The model under review builds one solid part; all positions refer to its coordinate system, in mm. A direction names the side the tool comes from. Coordinates: 2 decimals unless noted, no trailing zeros. Loops run counter-clockwise (first coordinate to the right, second up) from the corner with the lowest first, then second, coordinate; pieces in that order, holes last. Notation, with made-up numbers: M 64,68 L 71,68 A20 cw 71,93 Z; hole C 23,-18 d2. An arc over 180 degrees is marked long. Return JSON: item names as keys, results as strings.
Autodesk Fusion 360 part; units mm, degrees
sketch "スケッチ1" plane through (0, 0, 0) normal (0, 0, 1) x (1, 0, 0)
  line L0 (-19, 20) -> (19, 20)
  line L1 (19, 20) -> (19, 0)
  line L2 (19, 0) -> (-19, 0)
  line L3 (-19, 0) -> (-19, 20)
  dimension "d1" = 38
  dimension "d2" = 20
extrude "押し出し1" add sketch "スケッチ1" along normal blind 16
sketch "スケッチ2" plane through (0, 0, 16) normal (0, 0, 1) x (-1, 0, 0)
  line L0 (19, 0) -> (-19, 0)
  line L1 (-19, 0) -> (-19, -20)
  line L2 (-19, -20) -> (19, -20)
  line L3 (19, -20) -> (19, 0)
  line L4 (8, 0) -> (-8, 0)
  line L5 (-8, 0) -> (-8, -10)
  line L6 (-8, -10) -> (-15, -10)
  line L7 (-15, -10) -> (-15, -20)
  line L8 (15, -20) -> (15, -10)
  line L9 (15, -10) -> (8, -10)
  line L10 (8, -10) -> (8, 0)
  line L11 (14, -6) -> (-14, -6)
  point P0 (0, -6)
  dimension "d5" = 16
  dimension "d6" = 4
  dimension "d7" = 4
  dimension "d8" = 10
  dimension "d9" = 6
  dimension "d10" = 28
extrude "押し出し2" cut sketch "スケッチ2" against normal blind 11.5 contours L0 L4 L5 L10 L11 | L2 L5 L6 L7 L8 L9 L10 L11
hole "穴1" at (-14, 6, 16) at (14, 6, 16) direction (0, 0, -1) diameter 3 depth 10 tip angle 118
thread "ねじ1"
fillet "フィレット1" radius 4 2 edges at (19, 0, 8) (-19, 0, 8)
1. Add section A-A on y = 11.25. Give the boundary of the cut face in (x, z).
Check values:
{"outline": "M -19,0 L 19,0 L 19,16 L 15,16 L 15,4.5 L -15,4.5 L -15,16 L -19,16 Z"}
2. To check wall thickness, follow line 1 (X direction, y = 6, z = 10.25); line 2 (Y direction, x = 14, z = 10.5); line 3 (X direction, y = 8.75, z = 9.75). State the ranges of each line that lie inside material, in increasing order.
Check values:
{"line 1": "-19 to -15.5, -12.5 to -8, 8 to 12.5, 15.5 to 19", "line 2": "0 to 4.5, 7.5 to 10", "line 3": "-19 to -8, 8 to 19"}
3. The part is to be moulded in two halves that separate along Y. For faces 4 (the face through (14.22, 5.86, 5.255)), 5 (the face through (-13.1, 7.2, 10.9)), 6 (the face through (-12, 10, 10)), 7 (the face through (15, 8, 16)), say which applies: released by +Y, released by -Y, zero draft, split by the parting line, or undercut.
Check values:
{"face 4": "undercut", "face 5": "undercut", "face 6": "released by +Y", "face 7": "zero draft"}
4. Insertion check: pin 1 Ø7.5 at (x, z) = (11, 10.5) entering from +Y; pin 2 Ø6 at (x, y) = (7, 14.5) entering from +Z. Each pin has a flat end and moves straight along its axis. Give the tip position at first contact, or say it passes through.
Check values:
{"pin 1": "y = 10", "pin 2": "z = 4.5"}
5. Machinability: for faces 1 (the face through (-17.859, 1.203, 8.112)), 2 (the face through (8, 5, 10)), 3 (the face through (11, 10, 10)), which of the approach directions +Z, -Z, +X, -X, +Y, -Y give a long, thin tool a straight path to every point of the face, cutting with its end or side? Answer none if there is none.
Check values:
{"face 1": "+Z, -Z, -X, -Y", "face 2": "+Z, +Y, -Y", "face 3": "+Z, +Y"}
6. Add section B-B on x = -8.5. Give the boundary of the cut face in (y, z), plus the area to 3 significant figures.
Check values:
{"outline": "M 0,0 L 20,0 L 20,4.5 L 10,4.5 L 10,16 L 0,16 Z", "area": "205 mm²"}
